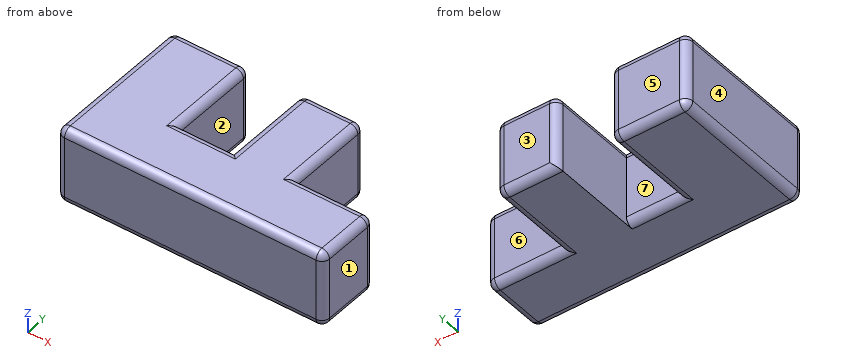
from build123d import *

# Parameters (mm, degrees)
BOSS_EXTRUDE2_DEPTH = 25.4
FILLET4_R           = 2.54
FILLET5_R           = 2.54
FILLET6_R           = 2.54


with BuildPart() as part:
    # Sketch1 → Boss-Extrude2 (new body)
    with BuildSketch(Plane.XY):
        Polygon((0, 0), (0, 50.8), (25.4, 50.8), (25.4, 20.561904762), (43.18, 20.561904762), (43.18, 50.8), (63.5, 50.8), (63.5, 21.59), (88.9, 21.59), (88.9, 0), align=None)
    extrude(amount=BOSS_EXTRUDE2_DEPTH)

    # Fillet4
    fillet4_edges = [part.edges().sort_by_distance(p)[0] for p in [
        (12.7, 50.8, 25.4),
    ]]
    fillet(fillet4_edges, radius=FILLET4_R)

    # Fillet5
    fillet5_edges = [part.edges().sort_by_distance(p)[0] for p in [
        (12.7, 50.8, 0),
        (25.4, 35.680952381, 0),
        (34.29, 20.561904762, 0),
        (53.34, 50.8, 0),
        (63.5, 36.195, 0),
        (76.2, 21.59, 25.4),
        (76.2, 21.59, 0),
        (63.5, 36.195, 25.4),
        (43.18, 50.8, 12.7),
        (63.5, 50.8, 12.7),
        (88.9, 21.59, 12.7),
        (53.34, 50.8, 25.4),
        (43.18, 35.680952381, 25.4),
        (34.29, 20.561904762, 25.4),
        (0, 24.13, 25.4),
        (0, 50.8, 11.43),
        (0, 50.056051224, 24.656051224),
        (25.4, 50.8, 11.43),
        (25.4, 50.056051224, 24.656051224),
        (25.4, 34.410952381, 25.4),
    ]]
    fillet(fillet5_edges, radius=FILLET5_R)

    # Fillet6
    # the kernel refuses this fillet: 2.54 mm, written as the material it takes off along each edge
    with BuildSketch(Plane(origin=(86.36, 19.05, 2.54), x_dir=(0, 0, -1), z_dir=(1, 0, 0))) as fillet6_piece_1_section:
        Polygon((0, 0), (FILLET6_R, 0), (FILLET6_R, FILLET6_R), (0, FILLET6_R), align=None)
    fillet6_piece_1 = extrude(amount=FILLET6_R, mode=Mode.PRIVATE)
    fillet6_piece_1 = fillet6_piece_1 - Plane(origin=(86.36, 19.05, 2.54), x_dir=(0, -0.7071067811865475, 0.7071067811865475), z_dir=(1, 0, 0)) * Sphere(FILLET6_R, mode=Mode.PRIVATE)
    add(fillet6_piece_1, mode=Mode.SUBTRACT)
    with BuildSketch(Plane(origin=(86.36, 19.05, 22.86), x_dir=(0, 0, 1), z_dir=(1, 0, 0))) as fillet6_piece_2_section:
        Polygon((0, 0), (FILLET6_R, 0), (FILLET6_R, -FILLET6_R), (0, -FILLET6_R), align=None)
    fillet6_piece_2 = extrude(amount=FILLET6_R, mode=Mode.PRIVATE)
    fillet6_piece_2 = fillet6_piece_2 - Plane(origin=(86.36, 19.05, 22.86), x_dir=(0, -0.7071067811865475, -0.7071067811865475), z_dir=(1, 0, 0)) * Sphere(FILLET6_R, mode=Mode.PRIVATE)
    add(fillet6_piece_2, mode=Mode.SUBTRACT)
    with BuildSketch(Plane(origin=(2.54, 48.26, 2.54), x_dir=(0, 0, -1), z_dir=(-1, 0, 0))) as fillet6_piece_3_section:
        Polygon((0, 0), (FILLET6_R, 0), (FILLET6_R, -FILLET6_R), (0, -FILLET6_R), align=None)
    fillet6_piece_3 = extrude(amount=FILLET6_R, mode=Mode.PRIVATE)
    fillet6_piece_3 = fillet6_piece_3 - Plane(origin=(2.54, 48.26, 2.54), x_dir=(0, -0.7071067811865475, 0.7071067811865475), z_dir=(-1, 0, 0)) * Sphere(FILLET6_R, mode=Mode.PRIVATE)
    add(fillet6_piece_3, mode=Mode.SUBTRACT)
    with BuildSketch(Plane(origin=(86.36, 2.54, 2.54), x_dir=(0, -1, 0), z_dir=(1, 0, 0))) as fillet6_piece_4_section:
        Polygon((0, 0), (FILLET6_R, 0), (FILLET6_R, FILLET6_R), (0, FILLET6_R), align=None)
    fillet6_piece_4 = extrude(amount=FILLET6_R, mode=Mode.PRIVATE)
    fillet6_piece_4 = fillet6_piece_4 - Plane(origin=(86.36, 2.54, 2.54), x_dir=(0, 0.7071067811865475, 0.7071067811865475), z_dir=(1, 0, 0)) * Sphere(FILLET6_R, mode=Mode.PRIVATE)
    add(fillet6_piece_4, mode=Mode.SUBTRACT)
    with BuildSketch(Plane(origin=(2.54, 2.54, 2.54), x_dir=(0, -1, 0), z_dir=(-1, 0, 0))) as fillet6_piece_5_section:
        Polygon((0, 0), (FILLET6_R, 0), (FILLET6_R, -FILLET6_R), (0, -FILLET6_R), align=None)
    fillet6_piece_5 = extrude(amount=FILLET6_R, mode=Mode.PRIVATE)
    fillet6_piece_5 = fillet6_piece_5 - Plane(origin=(2.54, 2.54, 2.54), x_dir=(0, 0.7071067811865475, 0.7071067811865475), z_dir=(-1, 0, 0)) * Sphere(FILLET6_R, mode=Mode.PRIVATE)
    add(fillet6_piece_5, mode=Mode.SUBTRACT)
    with BuildSketch(Plane(origin=(86.36, 2.54, 22.86), x_dir=(0, 0, 1), z_dir=(1, 0, 0))) as fillet6_piece_6_section:
        Polygon((0, 0), (FILLET6_R, 0), (FILLET6_R, FILLET6_R), (0, FILLET6_R), align=None)
    fillet6_piece_6 = extrude(amount=FILLET6_R, mode=Mode.PRIVATE)
    fillet6_piece_6 = fillet6_piece_6 - Plane(origin=(86.36, 2.54, 22.86), x_dir=(0, 0.7071067811865475, -0.7071067811865475), z_dir=(1, 0, 0)) * Sphere(FILLET6_R, mode=Mode.PRIVATE)
    add(fillet6_piece_6, mode=Mode.SUBTRACT)
    with BuildSketch(Plane(origin=(88.9, 19.05, 0), x_dir=(0, 0, 1), z_dir=(0, -1, 0))) as fillet6_piece_7:
        with BuildLine():
            CenterArc((FILLET6_R, FILLET6_R), FILLET6_R, 180, 90)
            Line((0, FILLET6_R), (0, 0))
            Line((0, 0), (FILLET6_R, 0))
        make_face()
    extrude(amount=16.51, mode=Mode.SUBTRACT)
    with BuildSketch(Plane(origin=(86.36, 0, 0), x_dir=(0, 0, 1), z_dir=(-1, 0, 0)), Plane(origin=(86.36, 0, 25.4), x_dir=(0, 1, 0), z_dir=(-1, 0, 0))) as fillet6_piece_8:
        with BuildLine():
            CenterArc((FILLET6_R, FILLET6_R), FILLET6_R, 180, 90)
            Line((0, FILLET6_R), (0, 0))
            Line((0, 0), (FILLET6_R, 0))
        make_face()
    extrude(amount=83.82, mode=Mode.SUBTRACT)
    with BuildSketch(Plane(origin=(88.9, 0, 2.54), x_dir=(0, 1, 0), z_dir=(0, 0, 1))) as fillet6_piece_9:
        with BuildLine():
            CenterArc((FILLET6_R, FILLET6_R), FILLET6_R, 180, 90)
            Line((0, FILLET6_R), (0, 0))
            Line((0, 0), (FILLET6_R, 0))
        make_face()
    extrude(amount=20.32, mode=Mode.SUBTRACT)
    with BuildSketch(Plane(origin=(0, 0, 2.54), x_dir=(0, 1, 0), z_dir=(0, 0, 1))) as fillet6_piece_10:
        with BuildLine():
            CenterArc((FILLET6_R, -FILLET6_R), FILLET6_R, 90, 90)
            Line((0, -FILLET6_R), (0, 0))
            Line((0, 0), (FILLET6_R, 0))
        make_face()
    extrude(amount=20.32, mode=Mode.SUBTRACT)
    with BuildSketch(Plane(origin=(2.54, 0, 22.86), x_dir=(-1, 0, 0), z_dir=(0, 0, -1))) as fillet6_piece_11:
        with BuildLine():
            CenterArc((2.54 - FILLET6_R, FILLET6_R), FILLET6_R, 270, 90)
            Line((2.54 - FILLET6_R, 0), (2.54, 0))
            Line((2.54, 0), (2.54, FILLET6_R))
        make_face()
    revolve(axis=Axis((2.54, 0, 22.86), (0, 1, 0)), revolution_arc=90, mode=Mode.SUBTRACT)
    with BuildSketch(Plane(origin=(0, 2.54, 0), x_dir=(0, 0, 1), z_dir=(0, 1, 0))) as fillet6_piece_12:
        with BuildLine():
            CenterArc((FILLET6_R, FILLET6_R), FILLET6_R, 180, 90)
            Line((0, FILLET6_R), (0, 0))
            Line((0, 0), (FILLET6_R, 0))
        make_face()
    extrude(amount=45.72, mode=Mode.SUBTRACT)
    with BuildSketch(Plane(origin=(88.9, 19.05, 25.4), x_dir=(0, 0, -1), z_dir=(0, -1, 0))) as fillet6_piece_13:
        with BuildLine():
            CenterArc((FILLET6_R, -FILLET6_R), FILLET6_R, 90, 90)
            Line((0, -FILLET6_R), (0, 0))
            Line((0, 0), (FILLET6_R, 0))
        make_face()
    extrude(amount=16.51, mode=Mode.SUBTRACT)


solid = part.part
Check sheet for the modelled part. Datum: model origin and axes. Units: mm. Face numbers are marked on the shaded views. A direction names the side the tool comes from. Coordinates: 2 decimals unless noted, no trailing zeros. Write each loop counter-clockwise with the first axis right and the second up, starting at its lowest first coordinate (ties: lowest second). Pieces come first, ordered by that corner, then holes.
Item 1: Scan lines: probe 1 along X at (y, z) = (46.5, 6.75); probe 2 along Y at (x, z) = (68.5, 13); probe 3 along X at (y, z) = (42, 23.5). Record each from-to range of solid material in increasing order.
Numbers:
probe 1: x = 0 to 25.4, 43.18 to 63.5
probe 2: y = 0 to 21.59
probe 3: x = 0.08 to 25.32, 43.26 to 63.42
Item 2: Cross-section at B-B on z = 7.75. Record the boundary of the cut face in (x, y).
Numbers:
outline: (0, 2.54) arc R2.54 ccw to (2.54, 0) - (86.36, 0) arc R2.54 ccw to (88.9, 2.54) - (88.9, 19.05) arc R2.54 ccw to (86.36, 21.59) - (63.5, 21.59) - (63.5, 48.26) arc R2.54 ccw to (60.96, 50.8) - (45.72, 50.8) arc R2.54 ccw to (43.18, 48.26) - (43.18, 20.56) - (25.4, 20.56) - (25.4, 48.26) arc R2.54 ccw to (22.86, 50.8) - (2.54, 50.8) arc R2.54 ccw to (0, 48.26) - close
Item 3: Depth check by flat-ended pin: pin 1 Ø6 at (x, z) = (72.5, 18) entering from +Y; pin 2 Ø12 at (y, z) = (30, 19) entering from +X; pin 3 Ø14 at (x, z) = (31, 15.5) entering from +Y; pin 4 Ø1 at (x, y) = (42, 31) entering from -Z. Enter the tip coordinate at first touch or a pass-through.
Numbers:
pin 1: stops at y = 21.59
pin 2: stops at x = 63.5
pin 3: stops at y = 50.53
pin 4: passes through
Item 4: Cross-section at C-C on x = 38. Record the boundary of the cut face in (y, z), then the cut area to 3 significant figures.
Numbers:
outline: (0, 2.54) arc R2.54 ccw to (2.54, 0) - (18.02, 0) arc R2.54 ccw to (20.56, 2.54) - (20.56, 22.86) arc R2.54 ccw to (18.02, 25.4) - (2.54, 25.4) arc R2.54 ccw to (0, 22.86) - close
area: 517 mm2
Item 5: Mould release check, pull along X, two halves, no side actions. Record for the marked faces 1, 2, 3 and 4: released by +X, released by -X, zero draft, split by the parting line, or undercut.
Numbers:
face 1: released by +X
face 2: undercut
face 3: zero draft
face 4: released by -X
Item 6: Cross-section at A-A on y = 30. Record the boundary of the cut face in (x, z).
Numbers:
outline: (0, 2.54) arc R2.54 ccw to (2.54, 0) - (22.86, 0) arc R2.54 ccw to (25.4, 2.54) - (25.4, 22.86) arc R2.54 ccw to (22.86, 25.4) - (2.54, 25.4) arc R2.54 ccw to (0, 22.86) - close; (43.18, 0) - (60.96, 0) arc R2.54 ccw to (63.5, 2.54) - (63.5, 22.86) arc R2.54 ccw to (60.96, 25.4) - (45.72, 25.4) arc R2.54 ccw to (43.18, 22.86) - close
Item 7: Access from +Z, -Z, +X, -X, +Y, -Y to the whole of each face (thin tool, end or side, straight path). Record for the marked faces 5, 6 and 7.
Numbers:
face 5: +Z, -Z, +X, -X, +Y
face 6: +Z, -Z, +X, +Y
face 7: +Z, -Z, +Y
Item 8: Cross-section at D-D on x = 65.5. Record the boundary of the cut face in (y, z).
Numbers:
outline: (0, 2.54) arc R2.54 ccw to (2.54, 0) - (19.05, 0) arc R2.54 ccw to (21.59, 2.54) - (21.59, 22.86) arc R2.54 ccw to (19.05, 25.4) - (2.54, 25.4) arc R2.54 ccw to (0, 22.86) - close
